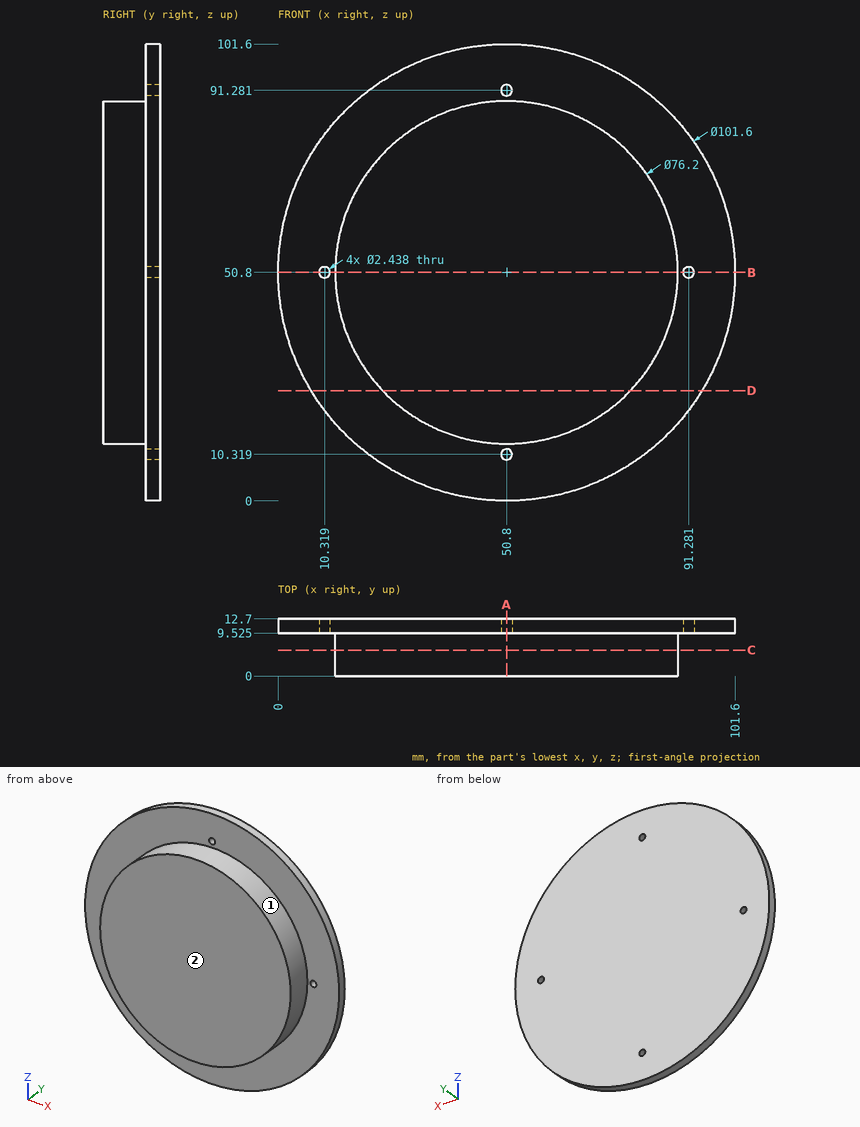
The drawing under review shows one solid part. Ordinate dimensions are in mm from its lowest x, y, z. A direction names the side the tool comes from. Give positions to 0.01 mm unless a question says otherwise; leave off trailing zeros. Loops run counter-clockwise (first coordinate to the right, second up) from the corner with the lowest first, then second, coordinate; pieces in that order, holes last. Notation, with made-up numbers: M 43.25,82.5 L 55.25,82.5 A14 ccw 55.25,105.5 Z; hole C 59,-36 d9. An arc over 180 degrees is marked long. One line per question, with ' | ' between items. Start each with the question number.
1. Add section C-C (y = 5.75). Write out the cut boundary in (x, z).
2. Add section A-A (x = 50.8). Write out the cut boundary in (y, z) (1 decimal).
3. Add section B-B (z = 50.8). Write out the cut boundary in (x, y) (1 decimal).
4. For the marked faces 1 and 2, list the 3-axis set-ups (+Z, -Z, +X, -X, +Y, -Y) from which the entire face can be reached by the end or side of a thin tool; tool diameter is ignored.
5. Insertion check: P1, Ø3, axis at x = 91.28, z = 50.8, coming from the -Y side (3 decimals). The pin has a flat end and moves straight along its axis. Give the tip position at first contact, or say it passes through.
6. To check wall thickness, follow L1, parallel to Y at x = 28.5, z = 91 (1 decimal); L2, parallel to X at y = 0.75, z = 51.5; L3, parallel to Z at x = 51, y = 7. State the ranges of each line that lie inside material, in increasing order.
7. Add section D-D (z = 24.5). Write out the cut boundary in (x, y) (1 decimal), plus the area to 3 significant figures.
Worked out:
1) outline: C 50.8,50.8 d76.2
2) outline: M 0,12.7 L 9.5,12.7 L 9.5,11.5 L 12.7,11.5 L 12.7,90.1 L 9.5,90.1 L 9.5,88.9 L 0,88.9 Z; M 9.5,0 L 12.7,0 L 12.7,9.1 L 9.5,9.1 Z; M 9.5,92.5 L 12.7,92.5 L 12.7,101.6 L 9.5,101.6 Z
3) outline: M 0,9.5 L 9.1,9.5 L 9.1,12.7 L 0,12.7 Z; M 11.5,9.5 L 12.7,9.5 L 12.7,0 L 88.9,0 L 88.9,9.5 L 90.1,9.5 L 90.1,12.7 L 11.5,12.7 Z; M 92.5,9.5 L 101.6,9.5 L 101.6,12.7 L 92.5,12.7 Z
4) face 1: -Y | face 2: +Z, -Z, +X, -X, -Y
5) P1: stops at y = 9.525
6) L1: y = 9.5 to 12.7 | L2: x = 12.71 to 88.89 | L3: z = 12.7 to 88.9
7) outline: M 7.3,9.5 L 23.2,9.5 L 23.2,0 L 78.4,0 L 78.4,9.5 L 94.3,9.5 L 94.3,12.7 L 7.3,12.7 Z | area: 801 mm²
